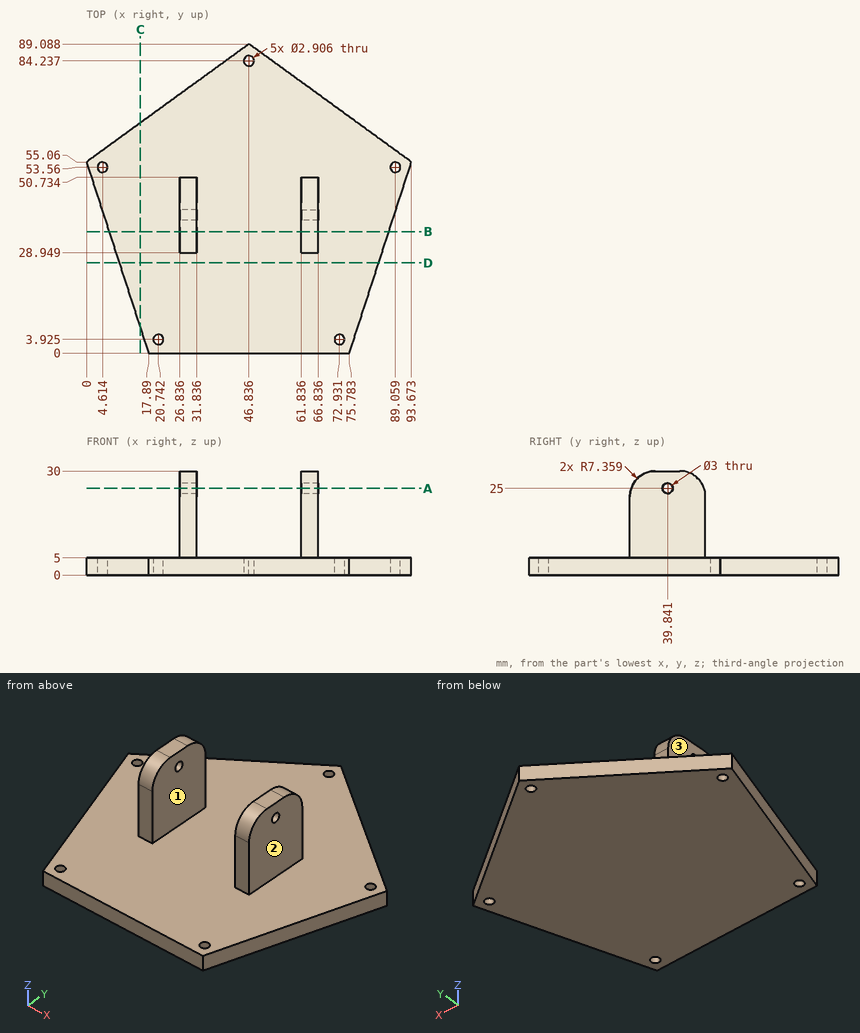
For this review, use the dimensioned drawing (mm, ordinates from the lowest corner) and the shaded views. Give positions to 0.01 mm unless a question says otherwise; leave off trailing zeros. Write each loop counter-clockwise with the first axis right and the second up, starting at its lowest first coordinate (ties: lowest second). Pieces come first, ordered by that corner, then holes.
(1) To check wall thickness, follow L1, parallel to X at y = 4.5, z = 3.25 (1 decimal); L2, parallel to Z at x = 12.5, y = 55; L3, parallel to X at y = 50.5, z = 22. State the ranges of each line that lie inside material, in increasing order.
(2) Consider section B-B, the plane y = 35. Give the boundary of the cut face in (x, z) (1 decimal).
(3) Consider section C-C, the plane x = 15.5. Give the boundary of the cut face in (y, z) (1 decimal).
(4) For P1, Ø1.5, axis at x = 28, z = 18, coming from the -Y side; P2, Ø6.5, axis at y = 40.5, z = 20, coming from the -X side; P3, Ø2.5, axis at x = 72.93, y = 3.93, coming from the -Z side; P4, Ø4, axis at x = 64, z = 15, coming from the +Y side, all flat-tipped, find the tip position at first contact; note any pin that passes through.
(5) Consider section D-D, the plane y = 26. Give the boundary of the cut face in (x, z).
(6) Consider section A-A, the plane z = 25. Give the boundary of the cut face in (x, y), and give its area (3 significant figures).
(7) The part is to be moulded in two halves that separate along X. For the marked faces 1, 2 and 3, say which applies: released by +X, released by -X, zero draft, split by the parting line, or undercut.
Returned:
1. L1: x = 16.4 to 19.4, 22.1 to 71.6, 74.3 to 77.2
1. L2: z = 0 to 5
1. L3: x = 26.84 to 31.84, 61.84 to 66.84
2. outline: (6.5, 0) - (87.2, 0) - (87.2, 5) - (66.8, 5) - (66.8, 29.9) - (61.8, 29.9) - (61.8, 5) - (31.8, 5) - (31.8, 29.9) - (26.8, 29.9) - (26.8, 5) - (6.5, 5) - close
3. outline: (7.4, 0) - (66.3, 0) - (66.3, 5) - (7.4, 5) - close
4. P1: stops at y = 28.95
4. P2: stops at x = 26.84
4. P3: passes through
4. P4: stops at y = 50.73
5. outline: (9.44, 0) - (84.23, 0) - (84.23, 5) - (9.44, 5) - close
6. outline: (26.84, 29.34) - (31.84, 29.34) - (31.84, 38.34) - (26.84, 38.34) - close; (26.84, 41.34) - (31.84, 41.34) - (31.84, 50.35) - (26.84, 50.35) - close; (61.84, 29.34) - (66.84, 29.34) - (66.84, 38.34) - (61.84, 38.34) - close; (61.84, 41.34) - (66.84, 41.34) - (66.84, 50.35) - (61.84, 50.35) - close
6. area: 180 mm2
7. face 1: undercut
7. face 2: released by +X
7. face 3: released by -X
